The listing builds one solid part. Answer for the finished solid, in the listing's coordinates (mm). A direction names the side the tool comes from. Give positions to 0.01 mm unless a question says otherwise; leave off trailing zeros. Order: outer loops, then holes, each group sorted by start corner. A loop starts at its lowest first (then second) coordinate and runs counter-clockwise, first axis right, second up. Notation, with made-up numbers: (64.25, 54.25) - (73.25, 54.25) arc R14 cw to (73.25, 70.25) - close; hole circle Ø4 at (49, -10). An arc over 180 degrees is marked (long way). Use CSV: the item, a comma, the result in double quotes.
```python
from build123d import *

# Parameters (mm, degrees)
PAD_DEPTH       = 4.5
POCKET_DEPTH    = 0.025
POCKET001_DEPTH = 0.025
SKETCH003_R     = 0.5
PAD001_DEPTH    = 0.175


with BuildPart() as part:
    # Sketch → Pad (new body, symmetric)
    with BuildSketch(Plane.XZ):
        with BuildLine():
            Line((0, 0), (0, 4))
            ThreePointArc((0.8, 4.8), (0.234315, 4.565685), (0, 4))
            Line((0.8, 4.8), (1.201873, 4.8))
            ThreePointArc((3.5, 2.501873), (2.826894, 4.126894), (1.201873, 4.8))
            Line((3.5, 2.501873), (3.5, -2))
            Line((3.5, -2), (3.8, -2))
            Line((3.8, 2), (3.8, -2))
            Line((3.7, 2), (3.8, 2))
            Line((3.7, 2.501873), (3.7, 2))
            ThreePointArc((3.7, 2.501873), (2.968316, 4.268316), (1.201873, 5))
            Line((0.8, 5), (1.201873, 5))
            ThreePointArc((0.8, 5), (0.092893, 4.707107), (-0.2, 4))
            Line((-0.2, 0), (-0.2, 4))
            Line((0, 0), (-0.2, 0))
        make_face()
    extrude(amount=PAD_DEPTH, both=True)

    # Sketch001 (on Face1 of Pad) → Pocket (cut)
    with BuildSketch(Plane(origin=(0, 0, 0), x_dir=(0, 0, 1), z_dir=(1, 0, 0))):
        Polygon((0, 3.818103), (2.005794, 3.818103), (2.005794, 3.318103), (0, 3.318103), (0, 2.818103), (2.005794, 2.818103), (2.005794, 2.318103), (0, 2.318103), (0, 1.818103), (2.005794, 1.818103), (2.005794, 1.318103), (0, 1.318103), (0, 0.818103), (2.005794, 0.818103), (2.005794, 0.318103), (0, 0.318103), (0, -0.181897), (2.005794, -0.181897), (2.005794, -0.681897), (0, -0.681897), (0, -1.181897), (2.005794, -1.181897), (2.005794, -1.681897), (0, -1.681897), (0, -2.181897), (2.005794, -2.181897), (2.005794, -2.681897), (0, -2.681897), (0, -3.181897), (2.005794, -3.181897), (2.005794, -3.681897), (0, -3.681897), (0, -4.5), (2.156164, -4.5), (2.156164, 4.5), (0, 4.5), align=None)
    extrude(amount=-POCKET_DEPTH, mode=Mode.SUBTRACT)

    # Sketch002 (on Face16 of Pocket) → Pocket001 (cut)
    with BuildSketch(Plane(origin=(3.5, 0, 0), x_dir=(0, 0, -1), z_dir=(-1, 0, 0))):
        Polygon((2, 3.749999), (-0.673578, 3.749999), (-0.673578, 3.249999), (2, 3.249999), (1.998494, 2.750001), (-0.675084, 2.750001), (-0.675084, 2.250001), (2, 2.250001), (2, 1.750001), (-0.673578, 1.750001), (-0.673578, 1.250001), (2, 1.250001), (2, 0.750001), (-0.673578, 0.750001), (-0.673578, 0.250001), (2, 0.250001), (2, -0.249999), (-0.673578, -0.249999), (-0.673578, -0.749999), (2, -0.749999), (2, -1.249999), (-0.673578, -1.249999), (-0.673578, -1.749999), (2, -1.749999), (2, -2.249999), (-0.673578, -2.249999), (-0.673578, -2.749999), (2, -2.749999), (2, -3.249999), (-0.673578, -3.249999), (-0.673578, -3.749999), (2, -3.749999), (2, -4.5), (-0.931806, -4.5), (-0.931806, 4.5), (2, 4.5), align=None)
    extrude(amount=-POCKET001_DEPTH, mode=Mode.SUBTRACT)

    # Sketch003 (on Face8 of Pocket001) → Pad001 (join)
    with BuildSketch(Plane(origin=(-0.2, 0, 0), x_dir=(0, 0, -1), z_dir=(-1, 0, 0))):
        Polygon((0, -4.5), (-0.5, -5.5), (-1, -6), (-2, -6), (-2.5, -5.5), (-3, -4.5), align=None)
        with Locations((-1.5, -5)):
            Circle(SKETCH003_R, mode=Mode.SUBTRACT)
        Polygon((0, 4.5), (-3, 4.5), (-2.5, 5.5), (-2, 6), (-1, 6), (-0.5, 5.5), align=None)
        with Locations((-1.5, 5)):
            Circle(SKETCH003_R, mode=Mode.SUBTRACT)
    extrude(amount=-PAD001_DEPTH)


solid = part.part
```
Item 1: The part is cut by section C-C (y = 0.5). Give the vertices of the cut face in (x, z) (3 decimals), and give its area (3 significant figures).
Taken from the geometry:
outline,"(-0.2, 0) - (0, 0) - (0, 2.006) - (-0.025, 2.006) - (-0.025, 2.156) - (0, 2.156) - (0, 4) arc R0.8 cw to (0.8, 4.8) - (1.202, 4.8) arc R2.298 cw to (3.5, 2.502) - (3.5, 0.932) - (3.525, 0.932) - (3.525, 0.674) - (3.5, 0.674) - (3.5, -2) - (3.8, -2) - (3.8, 2) - (3.7, 2) - (3.7, 2.502) arc R2.498 ccw to (1.202, 5) - (0.8, 5) arc R1 ccw to (-0.2, 4) - close"
area,"3.21 mm^2"
Item 2: The part is cut by section D-D (x = 1). Give the vertices of the cut face in (y, z).
Taken from the geometry:
outline,"(-4.5, 4.8) - (4.5, 4.8) - (4.5, 5) - (-4.5, 5) - close"
Item 3: Which of the six approach directions +Z, -Z, +X, -X, +Y, -Y give full straight-line access (tool end or side, diameter ignored) to faces 4 (the face through (3.8, 0, 0)), 5 (the face through (3.5, -2.42, -0.64))?
Taken from the geometry:
face 4,"+Z, -Z, +X, +Y, -Y"
face 5,"-Z, +Y, -Y"
Item 4: The part is cut by section B-B (y = -5). Give the vertices of the cut face in (x, z) (3 decimals), and give its area (4 significant figures).
Taken from the geometry:
outline,"(-0.2, 0.25) - (-0.025, 0.25) - (-0.025, 1) - (-0.2, 1) - close; (-0.2, 2) - (-0.025, 2) - (-0.025, 2.75) - (-0.2, 2.75) - close"
area,"0.2625 mm^2"
Item 5: Each of these flat-tipped pins is pushed along its axis until it touches: pin 1 (1.5 mm diameter, centred on x = 2, y = -3.5, fed in from -Z); pin 2 (1.5 mm diameter, centred on y = 1.5, z = 3.5, fed in from +X); pin 3 (1 mm diameter, centred on x = 1, y = 1, fed in from -Z). Where does it stop, or does it pass through?
Taken from the geometry:
pin 1,"z = 4.2"
pin 2,"x = 3.69"
pin 3,"z = 4.74"
Item 6: Find the intervals of material crossed by line 1 along X through (y, z) = (3.25, 0.75) (3 decimals); line 2 along Z through (x, y) = (-0.1, -5); line 3 along X through (y, z) = (2.5, -1.25), in increasing order.
Taken from the geometry:
line 1,"-0.2 to 0, 3.525 to 3.8"
line 2,"0.25 to 1, 2 to 2.75"
line 3,"3.5 to 3.8"
Item 7: The mould has two halves that part along X. Classify faces 1 (the face through (2.988, -0.063, 4.249)), 2 (the face through (-0.2, 0, 2)), 3 (the face through (2.845, -0.063, 4.109)): +X half, -X half, draft (parallel to the pull), parting line (faces both ways), or undercut.
Taken from the geometry:
face 1,"+X half"
face 2,"-X half"
face 3,"undercut"
Item 8: The part is cut by section A-A (z = 4.5). Give the vertices of the cut face in (x, y), and give its area (3 significant figures).
Taken from the geometry:
outline,"(-0.07, -4.5) - (0.18, -4.5) - (0.18, 4.5) - (-0.07, 4.5) - close; (2.34, -4.5) - (2.7, -4.5) - (2.7, 4.5) - (2.34, 4.5) - close"
area,"5.45 mm^2"
